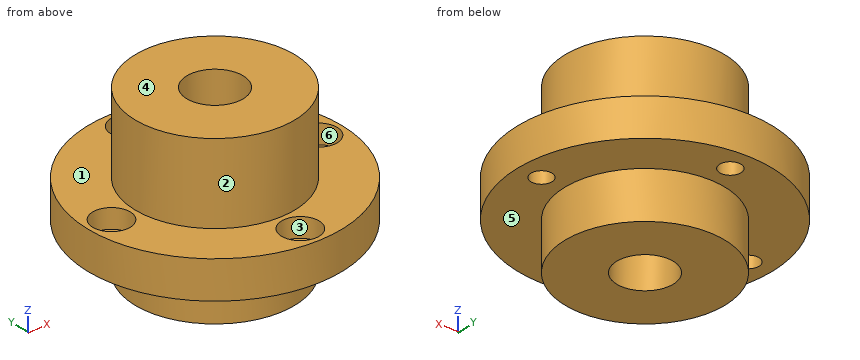
from build123d import *

# Parameters (mm, degrees)
F0_R           = 17
F0_R_2         = 6
F1_DEPTH       = 17
F2_R           = 27
F3_DEPTH       = 8
F4_R           = 17
F4_R_2         = 6
F5_DEPTH       = 10
F7_D           = 4.5
F7_CBORE_D     = 8
F7_CBORE_DEPTH = 4.1


with BuildPart() as f1:
    # F0 (on Top) → F1 (new body)
    with BuildSketch(Plane.XY):
        Circle(F0_R)
        Circle(F0_R_2, mode=Mode.SUBTRACT)
    extrude(amount=-F1_DEPTH)

    # F2 (on face) → F3 (join)
    with BuildSketch(Plane(origin=(0, 0, -17), x_dir=(1, 0, 0), z_dir=(0, 0, -1))):
        Circle(F2_R)
    extrude(amount=F3_DEPTH)

    # F4 (on face) → F5 (join)
    with BuildSketch(Plane(origin=(0, 0, -25), x_dir=(1, 0, 0), z_dir=(0, 0, -1))):
        Circle(F4_R)
        Circle(F4_R_2, mode=Mode.SUBTRACT)
    extrude(amount=F5_DEPTH)

    # F7 (through all)
    with Locations(Plane.XY.offset(-17)):
        with Locations((0, 22), (-22, 0), (0, -22), (22, 0)):
            CounterBoreHole(F7_D / 2, F7_CBORE_D / 2, F7_CBORE_DEPTH)


solid = f1.part
For this review, take the finished solid that the model builds, in its own axes (mm). Face numbers are marked on the shaded views. A direction names the side the tool comes from. Coordinates: 2 decimals unless noted, no trailing zeros. Order: outer loops, then holes, each group sorted by start corner. A loop starts at its lowest first (then second) coordinate and runs counter-clockwise, first axis right, second up. Notation, with made-up numbers: (42, -24.75) -> (56, -24.75) arc R18 cw to (56, 5.25) -> close; hole circle Ø9 at (17, -4.75). An arc over 180 degrees is marked (long way). Return JSON: item names as keys, results as strings.
1. We need section C-C on z = -15. Write out the cut boundary in (x, y).
Answer block:
{"outline": "circle Ø34 at (0, 0); hole circle Ø12 at (0, 0)"}
2. We need section A-A on x = 22. Write out the cut boundary in (y, z), and give its area (3 significant figures).
Answer block:
{"outline": "(-15.65, -25) -> (-2.25, -25) -> (-2.25, -21.1) -> (-4, -21.1) -> (-4, -17) -> (-15.65, -17) -> close; (2.25, -25) -> (15.65, -25) -> (15.65, -17) -> (4, -17) -> (4, -21.1) -> (2.25, -21.1) -> close", "area": "200 mm²"}
3. The part is to be moulded in two halves that separate along Y. For the marked faces 1, 2 and 3, say which applies: +Y half, -Y half, draft (parallel to the pull), parting line (faces both ways), or undercut.
Answer block:
{"face 1": "draft", "face 2": "parting line", "face 3": "undercut"}
4. We need section D-D on x = 16. Write out the cut boundary in (y, z).
Answer block:
{"outline": "(-21.75, -25) -> (-5.74, -25) -> (-5.74, -35) -> (5.74, -35) -> (5.74, -25) -> (21.75, -25) -> (21.75, -17) -> (5.74, -17) -> (5.74, 0) -> (-5.74, 0) -> (-5.74, -17) -> (-21.75, -17) -> close"}
5. For line 1 (Y direction, x = 0, z = -24.1); line 2 (Z direction, x = 21, y = -13.5); line 3 (X direction, y = -19.5, z = -18.5), list the stretches that pass through material, from the lowest coordinate up. Write a range as from..to.
Answer block:
{"line 1": "-27..-24.25, -19.75..19.75, 24.25..27", "line 2": "-25..-17", "line 3": "-18.67..-3.12, 3.12..18.67"}
6. Machinability: for the marked faces 4, 5 and 6, which of the approach directions +Z, -Z, +X, -X, +Y, -Y give a long, thin tool a straight path to every point of the face, cutting with its end or side? Answer none if there is none.
Answer block:
{"face 4": "+Z, +X, -X, +Y, -Y", "face 5": "-Z", "face 6": "+Z"}
7. For pin 1 Ø6 at (x, z) = (-8, -10.5) entering from +Y; pin 2 Ø6 at (x, y) = (2, 0) entering from +Z; pin 3 Ø5 at (x, z) = (-9, -31.5) entering from -Y, all flat-tipped, find the tip position at first contact; note any pin that passes through.
Answer block:
{"pin 1": "y = 16.25", "pin 2": "z = -17", "pin 3": "y = -15.71"}
